Could you check a few things on this model? Use its own coordinates, in mm. A direction names the side the tool comes from. Give positions to 0.01 mm unless a question says otherwise; leave off trailing zeros. Write each loop counter-clockwise with the first axis right and the second up, starting at its lowest first coordinate (ties: lowest second). Pieces come first, ordered by that corner, then holes. Notation, with made-up numbers: (79, 73) - (101, 73) arc R24 ccw to (101, 83) - close; hole circle Ø6 at (36.5, 84.5). An arc over 180 degrees is marked (long way). Answer in a Markdown table with one row per item.
Autodesk Fusion 360 part; units mm, degrees
sketch "Boceto9" plane through (0, 0, 0) normal (0, 0, 1) x (1, 0, 0)
  circle A0 centre (0, 0) radius 15
  dimension "d28" = 30
extrude "Extruir9" add sketch "Boceto9" along normal blind 4
sketch "Boceto10" plane through (0, 0, 4) normal (0, 0, 1) x (-1, 0, 0)
  circle A0 centre (0, 0) radius 15
  circle A1 centre (0, 0) radius 12.5
  dimension "d31" = 25
extrude "Extruir10" add sketch "Boceto10" along normal blind 4 contours A1
sketch "Boceto11" plane through (0, 0, 0) normal (0, 0, -1) x (1, 0, 0)
  circle A0 centre (0, 0) radius 15
  circle A1 centre (0, 0) radius 12.5
  circle A2 centre (0, 0) radius 7
  line L0 (0, 0) -> (-6.0622, 3.5)
  line L1 (0, 0) -> (7, 0) construction
  line L2 (0, 0) -> (6.0622, 3.5)
  line L3 (0, 0) -> (7, 0) construction
  line L4 (0, 0) -> (0, -7)
  circle A3 centre (6.0622, 3.5) radius 3.75
  circle A4 centre (-6.0622, 3.5) radius 3.75
  circle A5 centre (0, -7) radius 3.75
  circle A6 centre (6.0622, 3.5) radius 2
  circle A7 centre (-6.0622, 3.5) radius 2
  circle A8 centre (0, -7) radius 2
  dimension "d34" = 25
  dimension "d35" = 14
  dimension "d36" = 150
  dimension "d37" = 30
  dimension "d38" = 7
  dimension "d39" = 7.5
  dimension "d40" = 7.5
  dimension "d41" = 7.5
  dimension "d42" = 4
  dimension "d43" = 4
  dimension "d44" = 4
extrude "Extruir11" cut sketch "Boceto11" against normal blind 3 contours A2 L2 A3 A6 | A2 A3 A6 | A2 L2 A6 | A2 A6 | A2 L2 A6 | A2 L2 A3 A6 | A2 A5 A8 | A2 L4 A5 A8 | A2 A8 | A2 L4 A8 | A2 L4 A5 A8 | A2 L4 A8 | A2 L0 A4 A7 | A2 L0 A4 A7 | A2 A4 A7 | A2 L0 A7 | A2 L0 A7 | A2 A7
extrude "Extruir12" add 1 faces at (-0.3737, -9.0198, 0) along direction (0, 0, -1) blind 1
extrude "Extruir13" cut sketch "Boceto11" against normal blind 20 contours A2 L2 A6 | A2 A6 | A2 L2 A6 | A2 A8 | A2 L4 A8 | A2 L4 A8 | A2 L0 A7 | A2 L0 A7 | A2 A7
sketch "Boceto12" plane through (0, 0, 8) normal (0, 0, 1) x (-1, 0, 0)
  circle A0 centre (-6.0622, 3.5) radius 2
  circle A1 centre (6.0622, 3.5) radius 2
  circle A2 centre (0, -7) radius 2
  circle A3 centre (0, 0) radius 12.5
  circle A4 centre (0, 0) radius 2.8
  dimension "d51" = 5.6
extrude "Extruir14" add sketch "Boceto12" along normal blind 3.6 contours A4
move_face "CarasDesfase2" offset 0.15 3 faces at (-4.0721, -3.3009, 4.6667) (8.0522, -3.3009, 4.6667) (1.9901, 7.1991, 4.6667)
move_face "CarasDesfase3" offset 3 1 faces at (14.9814, -0.7477, 0.6667)
move_face "CarasDesfase4" offset 2 1 faces at (17.9776, -0.8972, 0.6667)
1) Imagine slicing it at A-A (x = 6). List the corners of the cut face in (y, z) for me.
Check values:
| item | result |
|---|---|
| outline | (-19.08, -1) - (-7.25, -1) - (-7.25, 3) - (-5.35, 3) - (-5.35, 8) - (-10.97, 8) - (-10.97, 4) - (-19.08, 4) - close; (-1.65, 3) - (0.25, 3) - (0.25, -1) - (19.08, -1) - (19.08, 4) - (10.97, 4) - (10.97, 8) - (-1.65, 8) - close |
2) On a 3-axis mill with a long thin cutter (end or side, diameter ignored), from which of +Z, -Z, +X, -X, +Y, -Y can I reach the whole of each face in a straight line? I mean faces 1 (the face through (-4.336, -19.524, 1.535)), 2 (the face through (9, 9, 4)), 3 (the face through (4, -3, 3)). Say none if no direction works.
Check values:
| item | result |
|---|---|
| face 1 | +Z, -Z |
| face 2 | +Z |
| face 3 | -Z |
3) If I drill on line 1 (Y direction, x = 0, z = 0.85); line 2 (X direction, y = -3.5, z = 5.65); line 3 (Z direction, x = 17, y = -3), over which ranges is the centre line in solid material (lowest first)?
Check values:
| item | result |
|---|---|
| line 1 | y = -20 to 3.25, 10.75 to 20 |
| line 2 | x = -12 to -7.91, -4.21 to 4.21, 7.91 to 12 |
| line 3 | z = -1 to 4 |
4) Will these pins go through, and if not, where does the flat tip stop? P1, Ø6, axis at x = 0, y = 7, coming from the +Z side; P2, Ø3, axis at y = -6, z = 4, coming from the +X side; P3, Ø2, axis at x = 1, y = 8, coming from the -Z side.
Check values:
| item | result |
|---|---|
| P1 | stops at z = 8 |
| P2 | stops at x = 19.49 |
| P3 | stops at z = 3 |
5) Imagine slicing it at B-B (y = -12). List the corners of the cut face in (x, z) for me.
Check values:
| item | result |
|---|---|
| outline | (-16, -1) - (16, -1) - (16, 4) - (3.5, 4) - (3.5, 8) - (-3.5, 8) - (-3.5, 4) - (-16, 4) - close |
6) Imagine slicing it at D-D (z = 2.5). List the corners of the cut face in (x, y) for me.
Check values:
| item | result |
|---|---|
| outline | circle Ø40 at (0, 0); hole circle Ø7.5 at (-6.06, -3.5); hole circle Ø7.5 at (0, 7); hole circle Ø7.5 at (6.06, -3.5) |
7) Imagine slicing it at C-C (y = 7). List the corners of the cut face in (x, z) for me (3 decimals).
Check values:
| item | result |
|---|---|
| outline | (-18.735, -1) - (-3.75, -1) - (-3.75, 3) - (-1.85, 3) - (-1.85, 8) - (-10.356, 8) - (-10.356, 4) - (-18.735, 4) - close; (1.85, 3) - (3.75, 3) - (3.75, -1) - (18.735, -1) - (18.735, 4) - (10.356, 4) - (10.356, 8) - (1.85, 8) - close |
8) We'd pull the mould along X, two halves only. Please class faces 4 (the face through (2.8, 0.1, 9.8)), 5 (the face through (0, 0, 11.6)), 6 (the face through (9.639, -2.374, 1.028)), 7 (the face through (-0.241, 5.166, 5.465)): +X half, -X half, draft (parallel to the pull), parting line (faces both ways), or undercut.
Check values:
| item | result |
|---|---|
| face 4 | parting line |
| face 5 | draft |
| face 6 | undercut |
| face 7 | undercut |
